Model file for the job. Use its own axes, mm. Face numbers are marked on the shaded views. A direction names the side the tool comes from. Give positions to 0.01 mm unless a question says otherwise; leave off trailing zeros. Answer in a Markdown table with one row per item.
```python
from build123d import *

# Parameters (mm, degrees)
CUT_EXTRUDE1_DEPTH = 7
SKETCH4_R          = 1.5
CUT_EXTRUDE2_DEPTH = 8.5
CHAMFER1_SIZE      = 0.5
FILLET1_R          = 0.5


with BuildPart() as part:
    # Sketch1 → Revolve1 (revolve)
    with BuildSketch(Plane.XY):
        with BuildLine():
            Line((3.5, 3.528396461), (3.5, 0))
            Line((3.5, 0), (9, 0))
            add(Edge.make_bspline(
                [(0, 23), (0.037336166, 22.983975753), (8.262108542, 21.480183495), (9, 0)],
                knots=[0, 0, 0, 0, 1, 1, 1, 1], degree=3))
            Line((0, 23), (0, 14))
            Line((0, 14), (3.5, 14))
            Line((3.5, 14), (3.5, 3.528396461))
        make_face()
    revolve(axis=Axis((0, 0, 0), (0, 1, 0)))

    # Sketch2 → Cut-Extrude1 (cut)
    with BuildSketch(Plane(origin=(0, 0, 0), x_dir=(1, 0, 0), z_dir=(0, 1, 0))):
        Polygon((5.629165125, 0), (2.814582562, 4.875), (-2.814582562, 4.875), (-5.629165125, 0), (-2.814582562, -4.875), (2.814582562, -4.875), align=None)
    extrude(amount=CUT_EXTRUDE1_DEPTH, mode=Mode.SUBTRACT)

    # Sketch4 → Cut-Extrude2 (cut, symmetric)
    with BuildSketch(Plane.XY):
        with Locations((0, 18)):
            Circle(SKETCH4_R)
    extrude(amount=CUT_EXTRUDE2_DEPTH, both=True, mode=Mode.SUBTRACT)

    # Chamfer1
    chamfer1_edges = [part.edges().sort_by_distance(p)[0] for p in [
        (4.221873843, 0, 2.4375),
        (4.221873843, 0, -2.4375),
        (0, 0, -4.875),
        (-4.221873843, 0, -2.4375),
        (-4.221873843, 0, 2.4375),
        (0, 0, 4.875),
    ]]
    chamfer(chamfer1_edges, length=CHAMFER1_SIZE)

    # Fillet1
    fillet1_edges = [part.edges().sort_by_distance(p)[0] for p in [
        (-3.5, 7, 0),
        (-3.5, 14, 0),
    ]]
    fillet(fillet1_edges, radius=FILLET1_R)


solid = part.part
```
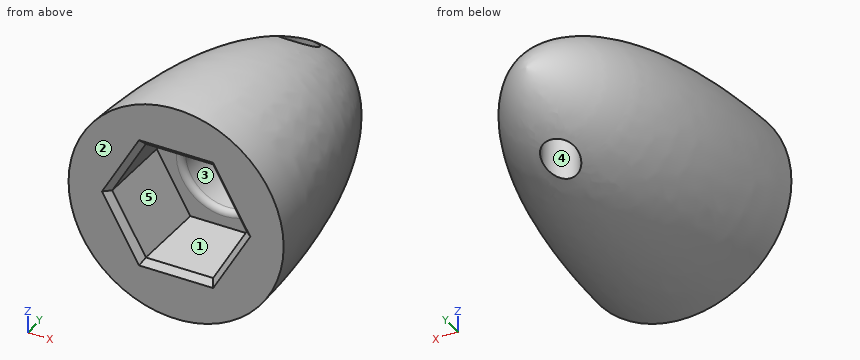
Q1. 3-axis set-ups, long thin cutter, end or side, ignore diameter. For the marked faces 4 and 5: which of +Z, -Z, +X, -X, +Y, -Y reach the whole face in a straight line?
Reported:
| item | result |
|---|---|
| face 4 | +Z, -Z |
| face 5 | -Y |
Q2. Drop flat-ended pins along their axis: pin 1 (8 mm diameter, centred on x = 0.5, z = 0, fed in from -Y); pin 2 (6 mm diameter, centred on x = -3, y = 5, fed in from -Z); pin 3 (1 mm diameter, centred on x = 0.5, y = 19, fed in from -Z). Give the stop position or say it passes through.
Reported:
| item | result |
|---|---|
| pin 1 | y = 7 |
| pin 2 | z = -8.81 |
| pin 3 | z = -4.41 |
Q3. Mould opens along Z. For the marked faces 1, 2 and 3 say: released by +Z, released by -Z, zero draft, split by the parting line, or undercut.
Reported:
| item | result |
|---|---|
| face 1 | undercut |
| face 2 | zero draft |
| face 3 | undercut |
Q4. Probe probe 1 along X at (y, z) = (5, 3); probe 2 along Z at (x, y) = (0, 9.85); probe 3 along Z at (x, y) = (-1.5, 9). List the from-to ranges inside material, lowest first.
Reported:
| item | result |
|---|---|
| probe 1 | -8.13 to -3.9, 3.9 to 8.13 |
| probe 2 | -7.95 to -3.5, 3.5 to 7.95 |
| probe 3 | -7.97 to -3.16, 3.16 to 7.97 |
